Can you work these out from the model? Positions are in its coordinate system, mm. A direction names the side the tool comes from. Give positions to 0.01 mm unless a question says otherwise; leave off trailing zeros. Loops run counter-clockwise (first coordinate to the right, second up) from the corner with the lowest first, then second, coordinate; pieces in that order, holes last. Notation, with made-up numbers: (7, 29.25) - (61, 29.25) arc R14 cw to (61, 50.25) - close; hole circle Ø1 at (28.25, 12). An arc over 180 degrees is marked (long way). Write item = value, one per line.
from build123d import *

# Parameters (mm, degrees)
BOSS_EXTRUDE1_DEPTH = 1.5
BOSS_EXTRUDE3_DEPTH = 20
LPATTERN1_COUNT     = 2
LPATTERN1_PITCH     = 40
SKETCH3_R           = 2.5
CUT_EXTRUDE1_DEPTH  = 20
CHAMFER1_SIZE       = 0.5


with BuildPart() as part:
    # Sketch1 → Boss-Extrude1 (new body)
    with BuildSketch(Plane(origin=(0, 0, 0), x_dir=(1, 0, 0), z_dir=(0, 1, 0))):
        with BuildLine():
            Line((-35, 17.5), (35, 17.5))
            ThreePointArc((35, 17.5), (38.535533906, 16.035533906), (40, 12.5))
            Line((40, 12.5), (40, -17.5))
            Line((40, -17.5), (-40, -17.5))
            Line((-40, -17.5), (-40, 12.5))
            ThreePointArc((-40, 12.5), (-38.535533906, 16.035533906), (-35, 17.5))
        make_face()
    extrude(amount=BOSS_EXTRUDE1_DEPTH)

    # Sketch2 → Boss-Extrude3 (add)
    with BuildSketch(Plane(origin=(40, 0, 0), x_dir=(0, 0, -1), z_dir=(1, 0, 0))):
        with BuildLine():
            Line((-17.5, 0), (-18.161538273, 0))
            ThreePointArc((-18.161538273, 0), (-25.221236665, 3.55341606), (-17.412973279, 2.329843428))
            Line((-17.412973279, 2.329843428), (-18.912973279, 2.329843428))
            ThreePointArc((-18.912973279, 2.329843428), (-23.877281896, 2.750774588), (-19.054719713, 1.5))
            Line((-19.054719713, 1.5), (-17.5, 1.5))
            Line((-17.5, 1.5), (-17.5, 0))
        make_face()
    boss_extrude3 = extrude(amount=-BOSS_EXTRUDE3_DEPTH)

    # LPattern1: Boss-Extrude3 ×2
    with Locations(*[(-i * LPATTERN1_PITCH, 0, 0) for i in range(1, LPATTERN1_COUNT)]):
        add(boss_extrude3)

    # Sketch3 → Cut-Extrude1 (cut)
    with BuildSketch(Plane(origin=(0, 1.5, 0), x_dir=(1, 0, 0), z_dir=(0, 1, 0))):
        with Locations(Location((0, 7.5, 0), (0, 0, 270))):
            Circle(SKETCH3_R)
        with Locations(Location((-26, -5.5, 0), (0, 0, 270))):
            Circle(SKETCH3_R)
        with Locations(Location((26, -5.5, 0), (0, 0, 270))):
            Circle(SKETCH3_R)
    extrude(amount=-CUT_EXTRUDE1_DEPTH, mode=Mode.SUBTRACT)

    # Chamfer1
    chamfer1_edges = [part.edges().sort_by_distance(p)[0] for p in [
        (0, 1.5, -10),
        (-26, 1.5, 3),
        (26, 1.5, 3),
    ]]
    chamfer(chamfer1_edges, length=CHAMFER1_SIZE)


solid = part.part
Q1. Imagine slicing it at B-B, the plane z = 5.5. Write out the boundary of the cut face in (x, y).
Output:
outline = (-40, 0) - (-28.5, 0) - (-28.5, 1) - (-29, 1.5) - (-40, 1.5) - close; (-23.5, 0) - (23.5, 0) - (23.5, 1) - (23, 1.5) - (-23, 1.5) - (-23.5, 1) - close; (28.5, 0) - (40, 0) - (40, 1.5) - (29, 1.5) - (28.5, 1) - close
Q2. We'd pull the mould along X, two halves only. Please class faces 6 (the cylindrical face through (28.11, 0.51, 6.84)), 7 (the flat face through (-20, -0.3, 22.2)), 8 (the cylindrical face through (-9.86, 3.402, 25.267)): released by +X, released by -X, zero draft, split by the parting line, or undercut.
Output:
face_6 = undercut
face_7 = released by -X
face_8 = zero draft
Q3. Imagine slicing it at D-D, the plane x = 33. Write out the boundary of the cut face in (y, z).
Output:
outline = (0, -17.5) - (1.5, -17.5) - (1.5, 19.05) arc R2.5 cw (long way) to (2.33, 18.91) - (2.33, 17.41) arc R4 ccw (long way) to (0, 18.16) - close
Q4. I need wall thicknesses on L1, parallel to X at y = 0.3, z = 5.5; L2, parallel to X at y = 0.55, z = -7.5; L3, parallel to X at y = 0, z = 23. Which ranges of each line are inside material? Lowest first, please.
Output:
L1 = -40 to -28.5, -23.5 to 23.5, 28.5 to 40
L2 = -40 to -2.5, 2.5 to 40
L3 = -20 to 0, 20 to 40
Q5. Imagine slicing it at C-C, the plane x = -26. Write out the boundary of the cut face in (y, z), then the cut area to 4 significant figures.
Output:
outline = (0, -17.5) - (1.5, -17.5) - (1.5, 2.5) - (1, 3) - (0, 3) - close; (0, 8) - (1, 8) - (1.5, 8.5) - (1.5, 17.5) - (0, 17.5) - close
area = 44.75 mm2
Q6. For pin 1 (18 mm diameter, centred on x = 14, z = -7.5, fed in from -Y); pin 2 (4 mm diameter, centred on y = 3, z = 20, fed in from -X); pin 3 (0.8 mm diameter, centred on x = 26, z = 18.5, fed in from -Y), each with a flat end and sliding along its axis, tell me the tip position at first contact or that it passes through.
Output:
pin_1 = 0
pin_2 = -20
pin_3 = -0.78
Q7. Imagine slicing it at A-A, the plane z = -7.5. Write out the boundary of the cut face in (x, y), then the cut area to 3 significant figures.
Output:
outline = (-40, 0) - (-2.5, 0) - (-2.5, 1) - (-3, 1.5) - (-40, 1.5) - close; (2.5, 0) - (40, 0) - (40, 1.5) - (3, 1.5) - (2.5, 1) - close
area = 112 mm2
Q8. Which directions (+Z, -Z, +X, -X, +Y, -Y) give clear straight access to the entire face, cutting with the end or side of a thin tool? Please do faces 1 (the flat face through (10, 1, 17.5)), 2 (the flat face through (0, 1, -17.5)), 3 (the flat face through (-30, 1, 17.5)), 4 (the cylindrical face through (30.14, 3.402, 25.267)), 5 (the flat face through (30, 2.33, 18)).
Output:
face_1 = +Z, +Y, -Y
face_2 = -Z, +X, -X, +Y, -Y
face_3 = +Z, -X, +Y, -Y
face_4 = +X, -X
face_5 = -Z, +X, -X
